Read the model definition and answer for the solid it produces. Units are mm, in the model's axes. Face numbers are marked on the shaded views. A direction names the side the tool comes from. Coordinates: 2 decimals unless noted, no trailing zeros. Loops run counter-clockwise (first coordinate to the right, second up) from the corner with the lowest first, then second, coordinate; pieces in that order, holes last. Notation, with made-up numbers: (-38.75, 14) - (-25.75, 14) arc R27 ccw to (-25.75, 39) - close; hole circle Ø7 at (38.5, 70). An arc over 180 degrees is marked (long way). Use one line per item in the form item = value. Start each with the question number.
1) A cutting plane is placed at D-D (z = 3.5). Give the vertices of the cut face in (x, y).
2) Each of these flat-tipped pins is pushed along its axis until it touches: P1, Ø8, axis at x = 61.5, z = 36.5, coming from the +Y side; P2, Ø12.5, axis at x = 6.5, z = 17, coming from the -Y side; P3, Ø2, axis at x = -12.5, y = -5.5, coming from the -Z side; P4, Ø6.5, axis at x = -8, z = 34.5, coming from the -Y side. Where does it stop, or does it pass through?
3) A cutting plane is placed at B-B (x = 54.5). Give the vertices of the cut face in (y, z), and give its area (3 significant figures).
4) A cutting plane is placed at A-A (z = 27.5). Give the vertices of the cut face in (x, y).
5) Consider line 1 (X direction, y = -4.5, z = 40); line 2 (Y direction, x = 74, z = 7); line 3 (Y direction, x = 68, z = 4.5). Determine where each line is inside the solid, lowest interval first.
6) A cutting plane is placed at C-C (y = 2.5). Give the vertices of the cut face in (x, z).
7) The mould has two halves that part along Y. Classify the marked faces 3, 4, 5 and 6: released by +Y, released by -Y, zero draft, split by the parting line, or undercut.
8) Which of the six approach directions +Z, -Z, +X, -X, +Y, -Y give full straight-line access (tool end or side, diameter ignored) to the marked faces 1 and 2?
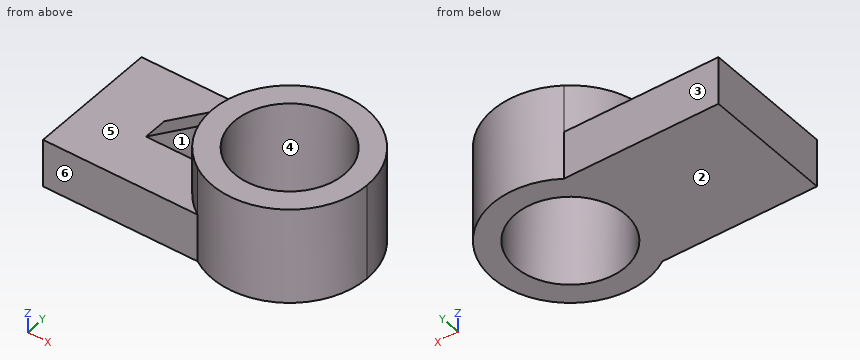
from build123d import *

# Parameters (mm, degrees)
F0_R     = 28.970038
F1_DEPTH = 50.8
F2_DEPTH = 25.4
F4_DEPTH = 6.35


with BuildPart() as f1:
    # F0 (on Top) → F1 (new body)
    with BuildSketch(Plane.XY):
        with BuildLine():
            ThreePointArc((92.899099, 0), (71.392782, 36.011503), (29.489314, 34.154247))
            ThreePointArc((29.489314, 34.154247), (11.092901, 0), (29.489314, -34.154247))
            ThreePointArc((29.489314, -34.154247), (71.392782, -36.011503), (92.899099, 0))
        make_face()
        with Locations((51.996, 0)):
            Circle(F0_R, mode=Mode.SUBTRACT)
    extrude(amount=F1_DEPTH)

    # F0 (on Top) → F2 (join)
    with BuildSketch(Plane.XY):
        with BuildLine():
            ThreePointArc((29.489314, -34.154247), (11.092901, 0), (29.489314, 34.154247))
            Line((29.489314, 34.154247), (-51.996, 34.154247))
            Line((-51.996, 34.154247), (-51.996, -34.154247))
            Line((-51.996, -34.154247), (29.489314, -34.154247))
        make_face()
        with BuildLine():
            ThreePointArc((92.899099, 0), (71.392782, 36.011503), (29.489314, 34.154247))
            ThreePointArc((29.489314, 34.154247), (11.092901, 0), (29.489314, -34.154247))
            ThreePointArc((29.489314, -34.154247), (71.392782, -36.011503), (92.899099, 0))
        make_face()
        with Locations((51.996, 0)):
            Circle(F0_R, mode=Mode.SUBTRACT)
    extrude(amount=F2_DEPTH)

    # F3 (on Front) → F4 (join, symmetric)
    with BuildSketch(Plane.XZ):
        Polygon((-25.342142, 20.81975), (10.89422, 20.81975), (10.89422, 46.377778), align=None)
    extrude(amount=F4_DEPTH, both=True)


solid = f1.part
Found:
q1.outline = (-52, -34.15) - (29.49, -34.15) arc R40.9 ccw (long way) to (29.49, 34.15) - (-52, 34.15) - close; hole circle Ø57.94 at (52, 0)
q2.P1 = 40.53
q2.P2 = -34.15
q2.P3 = 0
q2.P4 = -6.35
q3.outline = (-40.83, 0) - (-28.86, 0) - (-28.86, 50.8) - (-40.83, 50.8) - close; (28.86, 0) - (40.83, 0) - (40.83, 50.8) - (28.86, 50.8) - close
q3.area = 1,220 mm^2
q4.outline = (-15.87, -6.35) - (10.89, -6.35) - (10.89, 6.35) - (-15.87, 6.35) - close; circle Ø81.81 at (52, 0); hole circle Ø57.94 at (52, 0)
q5.line_1 = 1.85 to 10.89, 11.34 to 23.38, 80.61 to 92.65
q5.line_2 = -34.48 to -18.84, 18.84 to 34.48
q5.line_3 = -37.64 to -24.15, 24.15 to 37.64
q6.outline = (-52, 0) - (23.13, 0) - (23.13, 50.8) - (11.17, 50.8) - (11.17, 25.4) - (10.89, 25.4) - (10.89, 46.38) - (-18.85, 25.4) - (-52, 25.4) - close; (80.86, 0) - (92.82, 0) - (92.82, 50.8) - (80.86, 50.8) - close
q7.face_3 = released by +Y
q7.face_4 = undercut
q7.face_5 = zero draft
q7.face_6 = released by -Y
q8.face_1 = +Z, -X, -Y
q8.face_2 = -Z, +X, -X, +Y, -Y
